The model under review builds one solid part; all positions refer to its coordinate system, in mm. A direction names the side the tool comes from. Round coordinates to 2 decimals unless told otherwise and drop trailing zeros. Loops run counter-clockwise (first coordinate to the right, second up) from the corner with the lowest first, then second, coordinate; pieces in that order, holes last. Notation, with made-up numbers: M 45,43 L 73,43 A28 ccw 73,65 Z; hole C 30,22 d11. An arc over 180 degrees is marked long. Use a Markdown table: item, result. Add a question column.
```python
from build123d import *

# Parameters (mm, degrees)
F1_DEPTH = 2


with BuildPart() as f1:
    # F0 (on Front) → F1 (new body)
    with BuildSketch(Plane.XZ):
        with BuildLine():
            Line((-9.898934, 0), (-14.998934, 0))
            ThreePointArc((-14.998934, 0), (-0.149018, -14.953076), (14.997, -0.3))
            Line((14.997, -0.3), (9.897, -0.3))
            Line((9.897, -0.3), (9.897, -1.8))
            Line((9.897, -1.8), (11.897, -1.8))
            Line((11.897, -1.8), (11.897, -3.7))
            Line((11.897, -3.7), (6.797, -3.7))
            ThreePointArc((6.797, -3.7), (-3.766304, -6.802364), (-6.723454, 3.802508))
            Line((-6.723454, 3.802508), (-11.898934, 3.8))
            Line((-11.898934, 3.8), (-11.898934, 1.9))
            Line((-11.898934, 1.9), (-9.898934, 1.9))
            Line((-9.898934, 1.9), (-9.898934, 0))
        make_face()
    extrude(amount=F1_DEPTH)


solid = f1.part
```
(1) Insertion check: pin 1 Ø1.2 at (y, z) = (-1.5, -1) entering from -X; pin 2 Ø0.6 at (y, z) = (-0.5, 0.5) entering from -X; pin 3 Ø0.6 at (y, z) = (-1, -3) entering from -X. Each pin has a flat end and moves straight along its axis. Give the tip position at first contact, or say it passes through.
(2) Draft analysis for pull direction X (two halves, no side actions). For faces 1 (the face through (-12, -1, 0)), 2 (the face through (-3.62, -0.99, -6.88)), 3 (the face through (-0.476, -0.986, -14.946)), state which applies: released by +X, released by -X, zero draft, split by the parting line, or undercut.
(3) To check wall thickness, follow probe 1 along X at (y, z) = (-0.7, -5); probe 2 along X at (y, z) = (-1.05, -0.5); probe 3 along Z at (x, y) = (10.5, -1.35). State the ranges of each line that lie inside material, in increasing order.
(4) For faces 4 (the face through (-11.899, -1, 3)), 5 (the face through (11.897, -1, -3)), 6 (the face through (-11, -1, 1.9)), list the 3-axis set-ups (+Z, -Z, +X, -X, +Y, -Y) from which the entire face can be reached by the end or side of a thin tool; tool diameter is ignored.
(5) Consider section D-D, the plane z = -12.25. Give the boundary of the cut face in (x, y).
(6) Consider section B-B, the plane z = -5. Give the boundary of the cut face in (x, y), then the cut area to 3 significant figures.
(7) Consider section C-C, the plane x = -10.75. Give the boundary of the cut face in (y, z).
Found:
| question | item | result |
|---|---|---|
| 1 | pin 1 | stops at x = -14.99 |
| 1 | pin 2 | stops at x = -9.9 |
| 1 | pin 3 | stops at x = -14.75 |
| 2 | face 1 | zero draft |
| 2 | face 2 | undercut |
| 2 | face 3 | split by the parting line |
| 3 | probe 1 | x = -14.12 to -5.95, 5.92 to 14.13 |
| 3 | probe 2 | x = -14.99 to -7.73, 9.9 to 14.99 |
| 3 | probe 3 | z = -10.67 to -3.7, -1.8 to -0.3 |
| 4 | face 4 | +Z, -X, +Y, -Y |
| 4 | face 5 | +Y, -Y |
| 4 | face 6 | -X, +Y, -Y |
| 5 | outline | M -8.59,-2 L 8.59,-2 L 8.59,0 L -8.59,0 Z |
| 6 | outline | M -14.12,-2 L -5.95,-2 L -5.95,0 L -14.12,0 Z; M 5.92,-2 L 14.13,-2 L 14.13,0 L 5.92,0 Z |
| 6 | area | 32.8 mm^2 |
| 7 | outline | M -2,-10.41 L 0,-10.41 L 0,0 L -2,0 Z; M -2,1.9 L 0,1.9 L 0,3.8 L -2,3.8 Z |
